Geometry check sheet. Reference: the model listing, model coordinates, mm. Coordinates: 2 decimals unless noted, no trailing zeros. Write each loop counter-clockwise with the first axis right and the second up, starting at its lowest first coordinate (ties: lowest second). Pieces come first, ordered by that corner, then holes. Notation, with made-up numbers: M -36.5,30.5 L -21.5,30.5 A17 ccw -21.5,36.5 Z; hole C 20.25,-2 d4. An arc over 180 degrees is marked long. Put each result on its own line as item: value. Start each with the question number.
1) Gauge pin test, flat ends, axial feed: pin 1 (1 mm diameter, centred on x = 1, y = 1.5, fed in from -Z); pin 2 (3.5 mm diameter, centred on y = 0, z = 30.5, fed in from +X). Record the tip position at first contact, or that the pin passes through.
2) Cross-section at C-C on x = 1.1. Record the cut outline in (y, z).
3) Cross-section at B-B on y = 0. Record the cut outline in (x, z).
4) Cross-section at A-A on z = 21. Record the cut outline in (x, y).
5) Scan lines: line 1 along Z through (x, y) = (1.1, 0); line 2 along Y through (x, z) = (0.6, -30.5); line 3 along Z through (x, y) = (1.35, 1.05). Record each from-to range of solid material in increasing order.
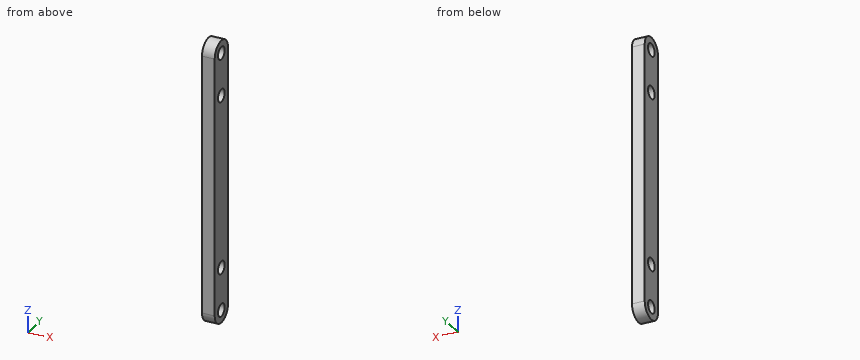
Autodesk Inventor part; units mm, degrees
ref_plane "YZ Plane" through (0, 0, 0) normal (1, 0, 0) x (0, 1, 0)
ref_plane "XZ Plane" through (0, 0, 0) normal (0, 1, 0) x (-1, 0, 0)
ref_plane "XY Plane" through (0, 0, 0) normal (0, 0, 1) x (1, 0, 0)
sketch "Sketch1" plane through (0, 0, 0) normal (1, 0, 0) x (0, 1, 0)
  line L0 (0, -30.5) -> (0, 30.5)
  line L1 (0, 20.422) -> (0, -20.422)
  circle A0 centre (0, 20.422) radius 1.5
  circle A1 centre (0, 30.5) radius 1.5
  circle A2 centre (0, -20.422) radius 1.5
  circle A3 centre (0, -30.5) radius 1.5
  line L2 (0, 30.5) -> (0, -30.5) construction
  line L3 (-3, 30.5) -> (-3, -30.5)
  line L4 (3, -30.5) -> (3, 30.5)
  arc A4 (3, 30.5) -> (-3, 30.5) centre (0, 30.5) ccw
  arc A5 (-3, -30.5) -> (3, -30.5) centre (0, -30.5) ccw
  point P0 (0, 0)
  point P1 (0, 0)
  dimension "d0" = 61
  dimension "d1" = 40.844
  dimension "d2" = 3
  dimension "d3" = 3
  dimension "d4" = 3
  dimension "d5" = 3
  dimension "d6" = 6
extrude "Extrusion1" add sketch "Sketch1" along normal blind 3
properties part number "wago_support_support"
Answer key:
1. pin 1: stops at z = -33.33
1. pin 2: stops at x = 3
2. outline: M -3,-30.5 A3 ccw 3,-30.5 L 3,30.5 A3 ccw -3,30.5 Z; hole C 0,-30.5 d3; hole C 0,-20.42 d3; hole C 0,20.42 d3; hole C 0,30.5 d3
3. outline: M 0,-33.5 L 3,-33.5 L 3,-32 L 0,-32 Z; M 0,-29 L 3,-29 L 3,-21.92 L 0,-21.92 Z; M 0,-18.92 L 3,-18.92 L 3,18.92 L 0,18.92 Z; M 0,21.92 L 3,21.92 L 3,29 L 0,29 Z; M 0,32 L 3,32 L 3,33.5 L 0,33.5 Z
4. outline: M 0,-3 L 3,-3 L 3,-1.38 L 0,-1.38 Z; M 0,1.38 L 3,1.38 L 3,3 L 0,3 Z
5. line 1: z = -33.5 to -32, -29 to -21.92, -18.92 to 18.92, 21.92 to 29, 32 to 33.5
5. line 2: y = -3 to -1.5, 1.5 to 3
5. line 3: z = -33.31 to -31.57, -29.43 to -21.49, -19.35 to 19.35, 21.49 to 29.43, 31.57 to 33.31
